Part model, mm, in its own coordinate system. Face numbers are marked on the shaded views. Round coordinates to 2 decimals unless told otherwise and drop trailing zeros. Loops run counter-clockwise (first coordinate to the right, second up) from the corner with the lowest first, then second, coordinate; pieces in that order, holes last.
Autodesk Inventor part; units mm, degrees
ref_plane "YZ Plane" through (0, 0, 0) normal (1, 0, 0) x (0, 1, 0)
ref_plane "XZ Plane" through (0, 0, 0) normal (0, 1, 0) x (-1, 0, 0)
ref_plane "XY Plane" through (0, 0, 0) normal (0, 0, 1) x (1, 0, 0)
sketch "Sketch1" plane through (0, 0, 0) normal (0, 0, 1) x (1, 0, 0)
  line L0 (0, 11.1125) -> (0, -11.1125)
  line L1 (-26.67, 0) -> (26.67, 0)
  line L2 (19.05, -7.9375) -> (-19.05, -7.9375)
  line L3 (-19.05, -7.9375) -> (-19.05, 7.9375)
  line L4 (-19.05, 7.9375) -> (19.05, 7.9375)
  line L5 (19.05, 7.9375) -> (19.05, -7.9375)
  line L6 (19.05, -7.9375) -> (-19.05, 7.9375) construction
  line L7 (-19.05, -7.9375) -> (19.05, 7.9375) construction
  point P0 (0, 0)
  point P1 (-12.7, 0)
  point P2 (12.7, 0)
  dimension "d0" = 38.1
  dimension "d1" = 12.7
  dimension "d2" = 12.7
  dimension "d3" = 15.875
extrude "Extrusion1" add sketch "Sketch1" against normal blind 6.35
hole "Hole1" at (-12.7, 0, 0) at (12.7, 0, 0) direction (0, 0, -1) diameter 4.4958 end through all countersink diameter 8.4328 countersink angle 100
fillet "Fillet1" radius 3.175 4 edges at (-19.05, 7.9375, -3.175) (19.05, 7.9375, -3.175) (19.05, -7.9375, -3.175) (-19.05, -7.9375, -3.175)
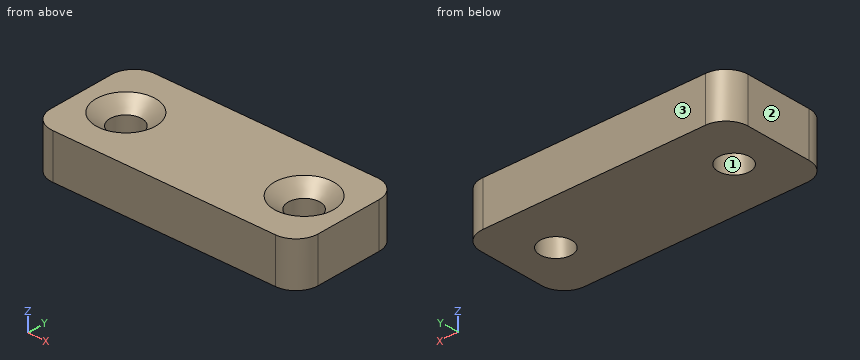
1) Drop a flat-ended pin along its axis: pin 1 Ø7 at (x, y) = (-12.7, 0) entering from +Z. Give the stop position or say it passes through.
Values:
pin 1: stops at z = -0.6
2) Wall check: line 1 along X through (y, z) = (0, -3.45); line 2 along Y through (x, z) = (-12.7, -5.05); line 3 along X through (y, z) = (1, -3). Give the ranges that are in metal, low to high.
Values:
line 1: x = -19.05 to -14.95, -10.45 to 10.45, 14.95 to 19.05
line 2: y = -7.94 to -2.25, 2.25 to 7.94
line 3: x = -19.05 to -14.71, -10.69 to 10.69, 14.71 to 19.05
3) Mould opens along Y. For the marked faces 1, 2 and 3 say: released by +Y, released by -Y, zero draft, split by the parting line, or undercut.
Values:
face 1: undercut
face 2: zero draft
face 3: released by +Y
4) Slice it at C-C, the plane y = 0. Give the cut face in (x, z).
Values:
outline: (-19.05, -6.35) - (-14.95, -6.35) - (-14.95, -1.65) - (-16.92, 0) - (-19.05, 0) - close; (-10.45, -6.35) - (10.45, -6.35) - (10.45, -1.65) - (8.48, 0) - (-8.48, 0) - (-10.45, -1.65) - close; (14.95, -6.35) - (19.05, -6.35) - (19.05, 0) - (16.92, 0) - (14.95, -1.65) - close
5) Slice it at A-A, the plane z = -4. Give the number of separate pieces and of enclosed holes in the cut face, then the cut area to 3 significant figures.
Values:
separate pieces: 1
enclosed holes: 2
area: 564 mm2
6) Slice it at B-B, the plane x = 12.7. Give the cut face in (y, z), then the cut area to 3 significant figures.
Values:
outline: (-7.94, -6.35) - (-2.25, -6.35) - (-2.25, -1.65) - (-4.22, 0) - (-7.94, 0) - close; (2.25, -6.35) - (7.94, -6.35) - (7.94, 0) - (4.22, 0) - (2.25, -1.65) - close
area: 69.0 mm2
